Check sheet for the modelled part. Datum: model origin and axes. Units: mm. A direction names the side the tool comes from. Round coordinates to 2 decimals unless told otherwise and drop trailing zeros. Write each loop counter-clockwise with the first axis right and the second up, starting at its lowest first coordinate (ties: lowest second). Pieces come first, ordered by that corner, then holes. Notation, with made-up numbers: (78.5, 17.25) -> (134.5, 17.25) arc R23 ccw to (134.5, 55.25) -> close; hole circle Ø2 at (86, 35.25). An arc over 180 degrees is marked (long way). Use one line per item in the form item = value. Start each with the question number.
```python
from build123d import *

# Parameters (mm, degrees)
SKETCH1_W                        = 100
SKETCH1_H                        = 100
BOSS_EXTRUDE1_DEPTH              = 16
CUT_EXTRUDE1_DEPTH               = 73.498275842
CUT_EXTRUDE1_DEPTH_BACK          = 73.498275842
SKETCH2_R                        = 23.5
SKETCH3_W                        = 1.85
SKETCH3_H                        = 1.75
TAP_DRILL_FOR_M6_HELICOIL1_D     = 6.25
TAP_DRILL_FOR_M6_HELICOIL1_DEPTH = 15
TAP_DRILL_FOR_M6_HELICOIL1_TIP   = 1.877689434
TAP_DRILL_FOR_M6_HELICOIL2_D     = 6.25
CHAMFER1_SIZE                    = 20


with BuildPart() as part:
    # Sketch1 → Boss-Extrude1 (new body)
    with BuildSketch(Plane.XY):
        Rectangle(SKETCH1_W, SKETCH1_H)
    extrude(amount=BOSS_EXTRUDE1_DEPTH)

    # Sketch2 → Cut-Extrude1 (cut, two sides: drawn at the far end of the back side and taken through both)
    with BuildSketch(Plane.XY.offset(16).offset(-CUT_EXTRUDE1_DEPTH_BACK)):
        Circle(SKETCH2_R)
    extrude(amount=CUT_EXTRUDE1_DEPTH + CUT_EXTRUDE1_DEPTH_BACK, mode=Mode.SUBTRACT)

    # Sketch3 → Cut-Revolve1 (revolve, cut)
    with BuildSketch(Plane(origin=(0, 0, 0), x_dir=(0, 0, -1), z_dir=(1, 0, 0)), mode=Mode.PRIVATE) as cut_revolve1_sk:
        with Locations((-12.925, 24.375)):
            Rectangle(SKETCH3_W, SKETCH3_H)
        with Locations((-3.075, 24.375)):
            Rectangle(SKETCH3_W, SKETCH3_H)
    revolve(cut_revolve1_sk.sketch.rotate(Axis((0, 0, 0), (0, 0, 1)), 90), axis=Axis((0, 0, 0), (0, 0, 1)), mode=Mode.SUBTRACT)

    # Tap Drill for M6 Helicoil1
    with Locations(Plane(origin=(0, -50, 0), x_dir=(-1, 0, 0), z_dir=(0, -1, 0))):
        with Locations((-40, -8), (0, -8), (40, -8)):
            Hole(TAP_DRILL_FOR_M6_HELICOIL1_D / 2, depth=TAP_DRILL_FOR_M6_HELICOIL1_DEPTH)
            with Locations((0, 0, -(TAP_DRILL_FOR_M6_HELICOIL1_DEPTH + TAP_DRILL_FOR_M6_HELICOIL1_TIP / 2))):  # 118° drill point
                Cone(0, TAP_DRILL_FOR_M6_HELICOIL1_D / 2, TAP_DRILL_FOR_M6_HELICOIL1_TIP, mode=Mode.SUBTRACT)

    # Tap Drill for M6 Helicoil2 (through all)
    with Locations(Plane(origin=(0, 0, 0), x_dir=(-1, 0, 0), z_dir=(0, 0, -1))):
        with Locations((-24.748737342, -24.748737342), (-24.748737342, 24.748737342), (24.748737342, 24.748737342), (24.748737342, -24.748737342)):
            Hole(TAP_DRILL_FOR_M6_HELICOIL2_D / 2)

    # Chamfer1
    chamfer1_edges = [part.edges().sort_by_distance(p)[0] for p in [
        (-50, 50, 8),
        (50, 50, 8),
    ]]
    chamfer(chamfer1_edges, length=CHAMFER1_SIZE)


solid = part.part
```
1. Sectioned sample at A-A (y = 0). Enter the section's corners in (x, z), and give its area (3 significant figures).
2. Sectioned sample at C-C (y = 32). Enter the section's corners in (x, z), and give its area (3 significant figures).
3. Depth check by flat-ended pin: pin 1 (5 mm diameter, centred on y = 40, z = 2.5, fed in from -X); pin 2 (4 mm diameter, centred on x = -40, z = 8, fed in from -Y); pin 3 (8 mm diameter, centred on x = 40, z = 8, fed in from +Y). Enter the tip coordinate at first touch or a pass-through.
4. Tool access check on faces 1 (the face through (24.342, 27.847, 8.112)), 2 (the face through (1.68, -42.395, 5.365)), 3 (the face through (20.04, 15.36, 3.06)). Record the directions out of +Z, -Z, +X, -X, +Y, -Y that give a thin tool (end or side, any length) a straight path to the whole face; none if there is none.
5. Sectioned sample at B-B (x = 16). Enter the section's corners in (y, z).
6. Mould release check, pull along X, two halves, no side actions. Record for faces 4 (the face through (40, 40, 8)), 5 (the face through (-37.02, -42.4, 7.06)), 6 (the face through (-1, -50, 4)), 7 (the face through (-25.43, -27.8, 8.11)): +X half, -X half, draft (parallel to the pull), parting line (faces both ways), or undercut.
7. Scan lines: probe 1 along Y at (x, z) = (0, 1.5); probe 2 along X at (y, z) = (26.5, 4.25); probe 3 along Y at (x, z) = (0, 3.35). Record each from-to range of solid material in increasing order.
Returned:
q1.outline = (-50, 0) -> (-23.5, 0) -> (-23.5, 2.15) -> (-25.25, 2.15) -> (-25.25, 4) -> (-23.5, 4) -> (-23.5, 12) -> (-25.25, 12) -> (-25.25, 13.85) -> (-23.5, 13.85) -> (-23.5, 16) -> (-50, 16) -> close; (23.5, 0) -> (50, 0) -> (50, 16) -> (23.5, 16) -> (23.5, 13.85) -> (25.25, 13.85) -> (25.25, 12) -> (23.5, 12) -> (23.5, 4) -> (25.25, 4) -> (25.25, 2.15) -> (23.5, 2.15) -> close
q1.area = 835 mm^2
q2.outline = (-48, 0) -> (48, 0) -> (48, 16) -> (-48, 16) -> close
q2.area = 1,540 mm^2
q3.pin_1 = -42.5
q3.pin_2 = -34.32
q3.pin_3 = 44
q4.face_1 = +Z, -Z
q4.face_2 = -Y
q4.face_3 = none
q5.outline = (-50, 0) -> (-17.21, 0) -> (-17.21, 2.15) -> (-19.53, 2.15) -> (-19.53, 4) -> (-17.21, 4) -> (-17.21, 12) -> (-19.53, 12) -> (-19.53, 13.85) -> (-17.21, 13.85) -> (-17.21, 16) -> (-50, 16) -> close; (17.21, 0) -> (50, 0) -> (50, 16) -> (17.21, 16) -> (17.21, 13.85) -> (19.53, 13.85) -> (19.53, 12) -> (17.21, 12) -> (17.21, 4) -> (19.53, 4) -> (19.53, 2.15) -> (17.21, 2.15) -> close
q6.face_4 = +X half
q6.face_5 = undercut
q6.face_6 = draft
q6.face_7 = undercut
q7.probe_1 = -50 to -23.5, 23.5 to 50
q7.probe_2 = -50 to -27.34, -22.16 to 22.16, 27.34 to 50
q7.probe_3 = -50 to -25.25, 25.25 to 50
